The listing builds one solid part. Answer for the finished solid, in the listing's coordinates (mm). A direction names the side the tool comes from. Round coordinates to 2 decimals unless told otherwise and drop trailing zeros. Write each loop counter-clockwise with the first axis right and the second up, starting at its lowest first coordinate (ties: lowest second). Pieces come first, ordered by that corner, then holes. Notation, with made-up numbers: (77.25, -4.75) - (106.25, -4.75) arc R27 ccw to (106.25, 24.25) - close; hole circle Ø11 at (-2.75, 76.5). An arc over 180 degrees is marked (long way). Return JSON: item names as keys, results as strings. Group by question number.
(1) Section C-C, the plane z = -37.5 is taken. Write down the section's boundary in (x, y).
(2) Determine the mould class of faces 5 (the flat face through (-14, 0, 0)), 6 (the flat face through (0, 24, -22)), 7 (the flat face through (0, 0, 0)) for opening direction Y: +Y half, -Y half, draft (parallel to the pull), parting line (faces both ways), or undercut.
(3) Each of these flat-tipped pins is pushed along its axis until it touches: pin 1 (13.5 mm diameter, centred on y = 8.5, z = -11.5, fed in from -X); pin 2 (5 mm diameter, centred on x = 2.5, z = -49, fed in from +Y); pin 3 (5 mm diameter, centred on x = 13.04, y = 0, fed in from +Z). Where does it stop, or does it pass through?
(4) Which of the six approach directions +Z, -Z, +X, -X, +Y, -Y give full straight-line access (tool end or side, diameter ignored) to faces 1 (the flat face through (13, 4, 7)), 2 (the cylindrical face through (15.62, 0.81, 9.01)), 3 (the flat face through (14, 0, 0)), 4 (the flat face through (-13, -4, 7))?
(5) Find the intervals of material crossed by line 1 along X through (y, z) = (0.5, -54); line 2 along Z through (x, y) = (-12.5, -6); line 3 along Y through (x, z) = (0, 3.25), in increasing order. Write a range as [from, to].
(6) Section B-B, the plane y = 0 is taken. Give the number of separate pieces and of enclosed holes in the cut face, then the cut area to 3 significant figures.
(7) Section A-A, the plane x = 0 is taken. Write down the section's boundary in (y, z), then the cut area to 3 significant figures.
```python
from build123d import *

# Parameters (mm, degrees)
ESQUISSE1_R                  = 17.5
BOSS_EXTRU_1_DEPTH           = 10
ESQUISSE3_W                  = 8
ESQUISSE3_H                  = 8
BOSS_EXTRU_3_DEPTH           = 4.5
ESQUISSE4_W                  = 2.5
ESQUISSE4_H                  = 8
ENL_V_MAT_EXTRU_1_DEPTH      = 1
ENL_V_MAT_EXTRU_1_DEPTH_BACK = 8
ESQUISSE5_R                  = 2.5
ENL_V_MAT_EXTRU_2_DEPTH      = 10.5
ESQUISSE6_W                  = 8
ESQUISSE6_H                  = 8
ESQUISSE6_R                  = 2.5
ENL_V_MAT_EXTRU_3_DEPTH      = 4.5
ESQUISSE7_W                  = 2.5
ESQUISSE7_H                  = 8
ENL_V_MAT_EXTRU_4_DEPTH      = 1
ENL_V_MAT_EXTRU_4_DEPTH_BACK = 8
ESQUISSE8_R                  = 2.707539361
ENL_V_MAT_EXTRU_5_DEPTH      = 10.5
ESQUISSE9_W                  = 8
ESQUISSE9_H                  = 8
ESQUISSE9_R                  = 2.707539361
ENL_V_MAT_EXTRU_6_DEPTH      = 4.5
ESQUISSE10_R                 = 5.5
ENL_V_MAT_EXTRU_7_DEPTH      = 11
ESQUISSE11_W                 = 24
ESQUISSE11_H                 = 48
BOSS_EXTRU_4_DEPTH           = 45
ESQUISSE12_R                 = 20
BOSS_EXTRU_5_DEPTH           = 13
ESQUISSE13_R                 = 11.5
ENL_V_MAT_EXTRU_8_DEPTH      = 8


with BuildPart() as part:
    # Esquisse1 → Boss.-Extru.1 (new body)
    with BuildSketch(Plane.XY):
        Circle(ESQUISSE1_R)
    extrude(amount=BOSS_EXTRU_1_DEPTH)

    # Esquisse3 → Boss.-Extru.3 (add)
    with BuildSketch(Plane.XY.offset(10)):
        with Locations((13.036725037, 0)):
            Rectangle(ESQUISSE3_W, ESQUISSE3_H)
        with Locations((-13.036725037, 0)):
            Rectangle(ESQUISSE3_W, ESQUISSE3_H)
    extrude(amount=BOSS_EXTRU_3_DEPTH)

    # Esquisse4 → Enlèv. mat.-Extru.1 (cut, two sides)
    with BuildSketch(Plane.ZY.offset(17.036725037)) as enl_v_mat_extru_1_sk:
        with Locations((6.75, 0)):
            Rectangle(ESQUISSE4_W, ESQUISSE4_H)
    extrude(amount=ENL_V_MAT_EXTRU_1_DEPTH, mode=Mode.SUBTRACT)
    extrude(enl_v_mat_extru_1_sk.sketch, amount=-ENL_V_MAT_EXTRU_1_DEPTH_BACK, mode=Mode.SUBTRACT)

    # Esquisse5 → Enlèv. mat.-Extru.2 (cut)
    with BuildSketch(Plane.XY.offset(14.5)):
        with Locations((-13.036725037, 0)):
            Circle(ESQUISSE5_R)
    extrude(amount=-ENL_V_MAT_EXTRU_2_DEPTH, mode=Mode.SUBTRACT)

    # Esquisse6 → Enlèv. mat.-Extru.3 (cut)
    with BuildSketch(Plane.XY.offset(14.5)):
        with Locations((-13.036725037, 0)):
            Rectangle(ESQUISSE6_W, ESQUISSE6_H)
        with Locations((-13.036725037, 0)):
            Circle(ESQUISSE6_R, mode=Mode.SUBTRACT)
    extrude(amount=-ENL_V_MAT_EXTRU_3_DEPTH, mode=Mode.SUBTRACT)

    # Esquisse7 → Enlèv. mat.-Extru.4 (cut, two sides)
    with BuildSketch(Plane(origin=(17.036725037, 0, 0), x_dir=(0, 0, -1), z_dir=(1, 0, 0))) as enl_v_mat_extru_4_sk:
        with Locations((-6.75, 0)):
            Rectangle(ESQUISSE7_W, ESQUISSE7_H)
    extrude(amount=ENL_V_MAT_EXTRU_4_DEPTH, mode=Mode.SUBTRACT)
    extrude(enl_v_mat_extru_4_sk.sketch, amount=-ENL_V_MAT_EXTRU_4_DEPTH_BACK, mode=Mode.SUBTRACT)

    # Esquisse8 → Enlèv. mat.-Extru.5 (cut)
    with BuildSketch(Plane.XY.offset(14.5)):
        with Locations((13.036725037, 0)):
            Circle(ESQUISSE8_R)
    extrude(amount=-ENL_V_MAT_EXTRU_5_DEPTH, mode=Mode.SUBTRACT)

    # Esquisse9 → Enlèv. mat.-Extru.6 (cut)
    with BuildSketch(Plane.XY.offset(14.5)):
        with Locations((13.036725037, 0)):
            Rectangle(ESQUISSE9_W, ESQUISSE9_H)
        with Locations((13.036725037, 0)):
            Circle(ESQUISSE9_R, mode=Mode.SUBTRACT)
    extrude(amount=-ENL_V_MAT_EXTRU_6_DEPTH, mode=Mode.SUBTRACT)

    # Esquisse10 → Enlèv. mat.-Extru.7 (cut, through all)
    with BuildSketch(Plane.XY.offset(10)):
        Circle(ESQUISSE10_R)
    extrude(amount=-ENL_V_MAT_EXTRU_7_DEPTH, mode=Mode.SUBTRACT)

    # Esquisse11 → Boss.-Extru.4 (add)
    with BuildSketch(Plane(origin=(0, 0, 0), x_dir=(-1, 0, 0), z_dir=(0, 0, -1))):
        Rectangle(ESQUISSE11_W, ESQUISSE11_H)
    extrude(amount=BOSS_EXTRU_4_DEPTH)

    # Esquisse12 → Boss.-Extru.5 (add)
    with BuildSketch(Plane(origin=(0, 0, -45), x_dir=(-1, 0, 0), z_dir=(0, 0, -1))):
        Circle(ESQUISSE12_R)
    extrude(amount=BOSS_EXTRU_5_DEPTH)

    # Esquisse13 → Enlèv. mat.-Extru.8 (cut)
    with BuildSketch(Plane(origin=(0, 0, -58), x_dir=(-1, 0, 0), z_dir=(0, 0, -1))):
        Circle(ESQUISSE13_R)
    extrude(amount=-ENL_V_MAT_EXTRU_8_DEPTH, mode=Mode.SUBTRACT)


solid = part.part
```
Working result:
{
 "1": {"outline": "(-12, -24) - (12, -24) - (12, 24) - (-12, 24) - close"},
 "2": {"face 5": "draft", "face 6": "+Y half", "face 7": "undercut"},
 "3": {"pin 1": "stops at x = -12", "pin 2": "stops at y = 20", "pin 3": "stops at z = 4"},
 "4": {"face 1": "+X", "face 2": "+Z", "face 3": "+X, +Y, -Y", "face 4": "-X"},
 "5": {"line 1": "x = [-19.99, -11.49], [11.49, 19.99]", "line 2": "z = [-58, -45], [0, 10]", "line 3": "y = [-17.5, -5.5], [5.5, 17.5]"},
 "6": {"separate pieces": "3", "enclosed holes": "0", "area": "1,580 mm^2"},
 "7": {"outline": "(-24, -45) - (-20, -45) - (-20, -58) - (-11.5, -58) - (-11.5, -50) - (11.5, -50) - (11.5, -58) - (20, -58) - (20, -45) - (24, -45) - (24, 0) - (17.5, 0) - (17.5, 10) - (5.5, 10) - (5.5, 0) - (-5.5, 0) - (-5.5, 10) - (-17.5, 10) - (-17.5, 0) - (-24, 0) - close", "area": "2,740 mm^2"}
}
